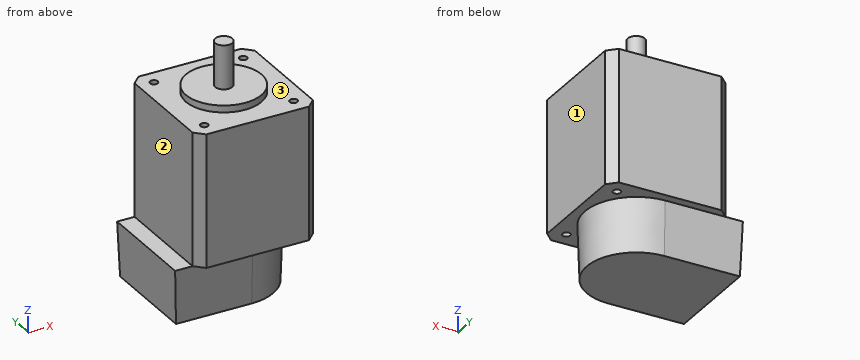
```python
from build123d import *

# Parameters (mm, degrees)
SKETCH1_W             = 35
SKETCH1_H             = 35
BOSS_EXTRUDE1_DEPTH   = 38.608
CHAMFER1_SIZE         = 2.54
SKETCH2_R             = 11.0236
BOSS_EXTRUDE2_DEPTH   = 2
SKETCH3_R             = 2.5
BOSS_EXTRUDE3_DEPTH   = 12.7
F_4_40_TAPPED_HOLE1_D = 2.2606
BOSS_EXTRUDE4_DEPTH   = 15.748
BOSS_EXTRUDE4_TAPER   = 2


with BuildPart() as part:
    # Sketch1 → Boss-Extrude1 (new body)
    with BuildSketch(Plane.XY):
        with Locations((17.5, 17.5)):
            Rectangle(SKETCH1_W, SKETCH1_H)
    extrude(amount=BOSS_EXTRUDE1_DEPTH)

    # Chamfer1
    chamfer1_edges = [part.edges().sort_by_distance(p)[0] for p in [
        (0, 35, 19.304),
        (35, 35, 19.304),
        (35, 0, 19.304),
        (0, 0, 19.304),
    ]]
    chamfer(chamfer1_edges, length=CHAMFER1_SIZE)

    # Sketch2 → Boss-Extrude2 (add)
    with BuildSketch(Plane.XY.offset(38.608)):
        with Locations(Location((17.5, 17.5, 0), (0, 0, 180))):  # turned: the seam where the file's is
            Circle(SKETCH2_R)
    extrude(amount=BOSS_EXTRUDE2_DEPTH)

    # Sketch3 → Boss-Extrude3 (add)
    with BuildSketch(Plane.XY.offset(40.608)):
        with Locations((17.5, 17.5)):
            Circle(SKETCH3_R)
    extrude(amount=BOSS_EXTRUDE3_DEPTH)

    # #4-40 Tapped Hole1 (through all)
    with Locations(Plane.XY.offset(38.608)):
        with Locations((4.5, 30.5), (30.5, 4.5), (4.5, 4.5), (30.5, 30.5)):
            Hole(F_4_40_TAPPED_HOLE1_D / 2)

    # Sketch6 → Boss-Extrude4 (add)
    with BuildSketch(Plane(origin=(0, 0, 0), x_dir=(-1, 0, 0), z_dir=(0, 0, -1))):
        with BuildLine():
            Line((5.08, 2.54), (5.08, 32.46))
            Line((5.08, 32.46), (-17.5, 32.46))
            ThreePointArc((-17.5, 32.46), (-32.46, 17.5), (-17.5, 2.54))
            Line((-17.5, 2.54), (5.08, 2.54))
        make_face()
    extrude(amount=BOSS_EXTRUDE4_DEPTH, taper=BOSS_EXTRUDE4_TAPER)


solid = part.part
```
Part model, mm, in its own coordinate system. Face numbers are marked on the shaded views. A direction names the side the tool comes from. Coordinates: 2 decimals unless noted, no trailing zeros. Order: outer loops, then holes, each group sorted by start corner. A loop starts at its lowest first (then second) coordinate and runs counter-clockwise, first axis right, second up. Notation, with made-up numbers: (72, 25.5) -> (96, 25.5) arc R25 ccw to (96, 53.5) -> close; hole circle Ø1 at (-21, 32). An arc over 180 degrees is marked (long way). Put each result on its own line as item: value. Start each with the question number.
(1) Band-saw the part on B-B (x = 30.5). Count the separate pieces of the cut face and the enclosed holes in it, then the cut area to 3 significant figures.
(2) Probe line 1 along Y through (x, z) = (4.5, 20.5); line 2 along Y through (x, z) = (30, 29); line 3 along Z through (x, y) = (25.5, 8). List the from-to ranges inside material, lowest first. Write a range as [from, to].
(3) Band-saw the part on A-A (z = 19). Give the cut face in (x, y), then the cut area to 3 significant figures.
(4) Pin check, flat tips, straight feed: pin 1 Ø1.8 at (x, y) = (30.5, 30.5) entering from +Z; pin 2 Ø5 at (y, z) = (27.5, 23.5) entering from -X; pin 3 Ø1.4 at (x, y) = (4.5, 30.5) entering from +Z; pin 4 Ø3 at (y, z) = (28, -4) entering from -X. Stop position of each tip, or through.
(5) Which spindle directions (+Z, -Z, +X, -X, +Y, -Y) get a long thin tool onto all of the face, cutting with end or side? Do the marked faces 1, 2 and 3. Say none if no direction does.
Determined:
1. separate pieces: 3
1. enclosed holes: 0
1. area: 1,390 mm²
2. line 1: y = [0, 3.37], [5.63, 29.37], [31.63, 35]
2. line 2: y = [0, 3.49], [5.51, 29.49], [31.51, 35]
2. line 3: z = [-15.75, 38.61]
3. outline: (0, 2.54) -> (2.54, 0) -> (32.46, 0) -> (35, 2.54) -> (35, 32.46) -> (32.46, 35) -> (2.54, 35) -> (0, 32.46) -> close; hole circle Ø2.26 at (4.5, 4.5); hole circle Ø2.26 at (4.5, 30.5); hole circle Ø2.26 at (30.5, 4.5); hole circle Ø2.26 at (30.5, 30.5)
3. area: 1,200 mm²
4. pin 1: passes through
4. pin 2: stops at x = 0
4. pin 3: stops at z = 0
4. pin 4: stops at x = -4.99
5. face 1: +Z, -Z, +X, +Y, -Y
5. face 2: +Z, -X, +Y, -Y
5. face 3: +Z
